from build123d import *

# Parameters (mm, degrees)
F3_D    = 6.35
F5_D    = 4.5
F6_SIZE = 0.79375


with BuildPart() as f1:
    # F0 (on Front) → F1 (revolve)
    with BuildSketch(Plane.XZ):
        with BuildLine():
            Line((0, 24), (0, 0))
            Line((0, 0), (22, 0))
            Line((22, 0), (22, 12))
            Line((22, 12), (5, 12))
            ThreePointArc((5, 12), (4.603125, 12.396875), (5, 12.79375))
            Line((5, 12.79375), (5, 24))
            Line((5, 24), (0, 24))
        make_face()
    revolve(axis=Axis((0, 0, 12), (0, 0, 1)))

    # F3 (through all)
    with Locations(Plane.XY.offset(24)):
        with Locations((0, 0)):
            Hole(F3_D / 2)

    # F5 (through all)
    with Locations(Plane.XY.offset(12)):
        with Locations((0, 14.5), (-14.5, 0), (0, -14.5), (14.5, 0)):
            Hole(F5_D / 2)

    # F6
    f6_edges = [f1.edges().sort_by_distance(p)[0] for p in [
        (-22, 0, 12),
        (-22, 0, 0),
        (22, 0, 6),
        (-5, 0, 24),
    ]]
    chamfer(f6_edges, length=F6_SIZE)


solid = f1.part
Geometry: final body of the model. Coordinates: model frame, mm. A direction names the side the tool comes from. Round coordinates to 2 decimals unless told otherwise and drop trailing zeros. Loops run counter-clockwise (first coordinate to the right, second up) from the corner with the lowest first, then second, coordinate; pieces in that order, holes last. Notation, with made-up numbers: M -7,44.25 L 40,44.25 A20 ccw 40,56.25 Z; hole C 31.5,41 d10. An arc over 180 degrees is marked long. Put each result on its own line as item: value. Start each with the question number.
(1) Section query A-A (y = 0). Return loops of the section in (x, z) (3 decimals), then the cut area to 3 significant figures.
(2) Material intervals for line 1 along Y through (x, z) = (0, 9.25) (3 decimals); line 2 along Z through (x, y) = (-11, -8); line 3 along Y through (x, z) = (-14.5, 7.75), sorted ascending. Write a range as [from, to].
(3) Contact query for flat-ended pins moving along their axis: pin 1 Ø1.5 at (y, z) = (11, 7.5) entering from -X; pin 2 Ø2 at (y, z) = (0, 20) entering from -X; pin 3 Ø8 at (x, z) = (7.5, 9.5) entering from +Y; pin 4 Ø4 at (x, y) = (0, -14.5) entering from +Z. Output: stop coordinate, or through.
(4) Section query C-C (z = 4.75). Return loops of the section in (x, y) (3 decimals), then the cut area to 3 significant figures.
(5) Set-up query: faces 4 (the face through (-2, 3, 24)), 5 (the face through (-1.08, -4.88, 18.07)). Return all of +Z, -Z, +X, -X, +Y, -Y with unobstructed straight access to the full face (end or side cutting, diameter ignored); none if empty.
(6) Draft query along X for faces 1 (the face through (-4.769, -21.477, 6.073)), 2 (the face through (0, -4, 0)), 3 (the face through (0.488, 12.304, 5.916)). Return one class per face: +X half, -X half, draft (parallel to the pull), parting line (faces both ways), or undercut.
(7) Section query D-D (z = 19.25). Return loops of the section in (x, y) (3 decimals).
Findings below:
1. outline: M -22,0.794 L -21.206,0 L -16.75,0 L -16.75,12 L -21.206,12 L -22,11.206 Z; M -12.25,0 L -3.175,0 L -3.175,24 L -4.206,24 L -5,23.206 L -5,12.794 A0.397 cw -5,12 L -12.25,12 Z; M 3.175,0 L 12.25,0 L 12.25,12 L 5,12 A0.397 cw 5,12.794 L 5,23.206 L 4.206,24 L 3.175,24 Z; M 16.75,0 L 21.206,0 L 22,0.794 L 22,11.206 L 21.206,12 L 16.75,12 Z
1. area: 385 mm2
2. line 1: y = [-22, -16.75], [-12.25, -3.175], [3.175, 12.25], [16.75, 22]
2. line 2: z = [0, 12]
2. line 3: y = [-16.55, -2.25], [2.25, 16.55]
3. pin 1: stops at x = -19.47
3. pin 2: stops at x = -5
3. pin 3: stops at y = 21.72
3. pin 4: passes through
4. outline: C 0,0 d44; hole C -14.5,0 d4.5; hole C 0,0 d6.35; hole C 0,-14.5 d4.5; hole C 0,14.5 d4.5; hole C 14.5,0 d4.5
4. area: 1,430 mm2
5. face 4: +Z, +X, -X, +Y, -Y
5. face 5: +Z
6. face 1: parting line
6. face 2: draft
6. face 3: undercut
7. outline: C 0,0 d10; hole C 0,0 d6.35
